```python
from build123d import *

# Parameters (mm, degrees)
SHELL1_T           = -2.8
SKETCH6_R          = 5.1
CUT_EXTRUDE4_DEPTH = 15


with BuildPart() as part:
    # Sketch1 → Revolve1 (revolve)
    with BuildSketch(Plane(origin=(0, 0, 0), x_dir=(1, 0, 0), z_dir=(0, 1, 0))):
        Polygon((0, 0), (-8, 0), (-8, -15), (-4, -23), (0, -23), align=None)
    revolve(axis=Axis((0, 0, -36.045977011), (0, 0, 1)))

    # Shell1
    shell1_openings = [part.faces().sort_by_distance(p)[0] for p in [
        (0, 0, 23),
    ]]
    offset(amount=SHELL1_T, openings=shell1_openings, kind=Kind.INTERSECTION)

    # Sketch6 → Cut-Extrude4 (cut)
    with BuildSketch(Plane(origin=(0, 0, 0), x_dir=(-1, 0, 0), z_dir=(0, 0, -1))):
        Circle(SKETCH6_R)
    extrude(amount=-CUT_EXTRUDE4_DEPTH, mode=Mode.SUBTRACT)


solid = part.part
```
Design review of the part built by this model. Coordinates are the model's own, in mm. A direction names the side the tool comes from. Give positions to 0.01 mm unless a question says otherwise; leave off trailing zeros. Order: outer loops, then holes, each group sorted by start corner. A loop starts at its lowest first (then second) coordinate and runs counter-clockwise, first axis right, second up. Notation, with made-up numbers: M 42,15.5 L 93,15.5 A30 cw 93,37.5 Z; hole C 85.5,-3.75 d10. An arc over 180 degrees is marked long. One line per question, with ' | ' between items. Start each with the question number.
Q1. We need section B-B (z = 1.5). Write out the cut boundary in (x, y).
Q2. We need section D-D (z = 10.25). Write out the cut boundary in (x, y), plus the area to 3 significant figures.
Q3. Machinability: for faces 1 (the face through (1.73, 7.81, 7.6)), 2 (the face through (-2.4, -4.5, 1.4)), 3 (the face through (0.677, -5.156, 8.65)), which of the approach directions +Z, -Z, +X, -X, +Y, -Y give a long, thin tool a straight path to every point of the face, cutting with its end or side? Answer none if there is none.
Q4. We need section A-A (y = 0). Write out the cut boundary in (x, z).
Q5. For pin 1 Ø4 at (x, z) = (6, 9) entering from -Y; pin 2 Ø3 at (x, y) = (-1, -0.5) entering from -Z; pin 3 Ø2 at (y, z) = (4, 3) entering from +X; pin 4 Ø4 at (x, y) = (5, 6.5) entering from -Z, all flat-tipped, find the tip position at first contact; note any pin that passes through.
Q6. The part is to be moulded in two halves that separate along X. For faces 4 (the face through (0.6, -4.6, 21.72)), 5 (the face through (5, 2, 0)), 6 (the face through (-2.4, -4.5, 14.8)), say which applies: +X half, -X half, draft (parallel to the pull), parting line (faces both ways), or undercut.
Q7. For L1, parallel to Y at x = 0, z = 1.2; L2, parallel to Y at x = 4.25, z = 2, list the stretches that pass through material, from the lowest coordinate up. Write a range as [from, to].
Returned:
1) outline: C 0,0 d16; hole C 0,0 d10.2
2) outline: C 0,0 d16; hole C 0,0 d10.4 | area: 116 mm2
3) face 1: +Z, -Z | face 2: -Z | face 3: none
4) outline: M -8,0 L -5.1,0 L -5.1,2.8 L -5.2,2.8 L -5.2,14.34 L -5.1,14.54 L -5.1,15 L -4.87,15 L -0.87,23 L -4,23 L -8,15 Z; M 0.87,23 L 4.87,15 L 5.1,15 L 5.1,14.54 L 5.2,14.34 L 5.2,2.8 L 5.1,2.8 L 5.1,0 L 8,0 L 8,15 L 4,23 Z
5) pin 1: y = -6.93 | pin 2: z = 19.5 | pin 3: x = 7.42 | pin 4: z = 0
6) face 4: parting line | face 5: draft | face 6: undercut
7) L1: [-8, -5.1], [5.1, 8] | L2: [-6.78, -2.82], [2.82, 6.78]
